For this review, take the finished solid that the model builds, in its own axes (mm). A direction names the side the tool comes from. Give positions to 0.01 mm unless a question says otherwise; leave off trailing zeros. Loops run counter-clockwise (first coordinate to the right, second up) from the corner with the lowest first, then second, coordinate; pieces in that order, holes last. Notation, with made-up numbers: (-24.75, 83.25) - (-1.75, 83.25) arc R29 cw to (-1.75, 116.25) - close; hole circle Ø11 at (66, 39.25). An arc over 180 degrees is marked (long way). Put each result on its own line as item: value.
from build123d import *

# Parameters (mm, degrees)
BOSS_EXTRUDE1_DEPTH = 3


with BuildPart() as part:
    # Sketch1 → Boss-Extrude1 (new body)
    with BuildSketch(Plane.XY):
        with BuildLine():
            ThreePointArc((-10.225, -10.225), (0, 0), (10.225, -10.225))
            Line((10.225, -10.225), (20.5, -10.225))
            Line((20.5, -10.225), (20.5, 10.225))
            Line((20.5, 10.225), (14.535, 10.225))
            Line((14.535, 10.225), (14.535, 13.225))
            Line((14.535, 13.225), (8.535, 13.225))
            Line((8.535, 13.225), (8.535, 10.225))
            Line((8.535, 10.225), (-8.535, 10.225))
            Line((-8.535, 10.225), (-8.535, 13.225))
            Line((-8.535, 13.225), (-14.535, 13.225))
            Line((-14.535, 13.225), (-14.535, 10.225))
            Line((-14.535, 10.225), (-20.5, 10.225))
            Line((-20.5, 10.225), (-20.5, -10.225))
            Line((-20.5, -10.225), (-10.225, -10.225))
        make_face()
    extrude(amount=BOSS_EXTRUDE1_DEPTH)


solid = part.part
1) For faces 5 (the face through (0, 10.225, 1)), 6 (the face through (18, 10.225, 1)), 7 (the face through (20.5, 0, 1)), list the 3-axis set-ups (+Z, -Z, +X, -X, +Y, -Y) from which the entire face can be reached by the end or side of a thin tool; tool diameter is ignored.
Geometry check:
face 5: +Z, -Z, +Y
face 6: +Z, -Z, +X, +Y
face 7: +Z, -Z, +X, +Y, -Y
2) Insertion check: pin 1 Ø0.9 at (y, z) = (11, 1.5) entering from -X (3 decimals); pin 2 Ø0.9 at (y, z) = (12.5, 1.5) entering from +X (3 decimals). Each pin has a flat end and moves straight along its axis. Give the tip position at first contact, or say it passes through.
Geometry check:
pin 1: stops at x = -14.535
pin 2: stops at x = 14.535
3) Take a section at B-B on x = -16.5. State the section outline as (y, z) points (3 decimals), and give its area (4 significant figures).
Geometry check:
outline: (-10.225, 0) - (10.225, 0) - (10.225, 3) - (-10.225, 3) - close
area: 61.35 mm²
4) Take a section at C-C on x = -5.5. State the section outline as (y, z) points (3 decimals), and give its area (3 significant figures).
Geometry check:
outline: (-1.605, 0) - (10.225, 0) - (10.225, 3) - (-1.605, 3) - close
area: 35.5 mm²
5) Take a section at A-A on z = 1.5. State the section outline as (x, y) points (3 decimals).
Geometry check:
outline: (-20.5, -10.225) - (-10.225, -10.225) arc R10.225 cw to (10.225, -10.225) - (20.5, -10.225) - (20.5, 10.225) - (14.535, 10.225) - (14.535, 13.225) - (8.535, 13.225) - (8.535, 10.225) - (-8.535, 10.225) - (-8.535, 13.225) - (-14.535, 13.225) - (-14.535, 10.225) - (-20.5, 10.225) - close
6) Draft analysis for pull direction X (two halves, no side actions). For faces 1 (the face through (-17, 10.225, 1)), 2 (the face through (-8.535, 12, 1)), 3 (the face through (-14.535, 12, 1)), 4 (the face through (0, 0, 1)), state which applies: pulls with the +X half, pulls with the -X half, needs draft (parallel to the pull), parting line crosses it, or undercut.
Geometry check:
face 1: needs draft
face 2: undercut
face 3: pulls with the -X half
face 4: undercut
7) Wall thickness on line 1 (X direction, y = -7.5, z = 2.1); line 2 (X direction, y = -4.5, z = 0.2); line 3 (Y direction, x = -6, z = 2.1) (3 decimals): over which ranges is each line inside the solid? List them lowest first.
Geometry check:
line 1: x = -20.5 to -9.86, 9.86 to 20.5
line 2: x = -20.5 to -8.47, 8.47 to 20.5
line 3: y = -1.945 to 10.225
